The listing builds one solid part. Answer for the finished solid, in the listing's coordinates (mm). Face numbers are marked on the shaded views. Coordinates: 2 decimals unless noted, no trailing zeros. Write each loop counter-clockwise with the first axis right and the second up, starting at its lowest first coordinate (ties: lowest second). Pieces come first, ordered by that corner, then holes. Notation, with made-up numbers: M 17.25,43 L 37.25,43 A15 cw 37.25,62 Z; hole C 54,-27.5 d2. An arc over 180 degrees is marked long. Answer as CSV lines item,"result". Start each with the question number.
```python
from build123d import *

# Parameters (mm, degrees)
F0_R     = 40.88
F0_R_2   = 2.1
F0_R_3   = 40
F1_DEPTH = 2
F2_DEPTH = 10


# Not quite as in the source:
# - a fillet or chamfer that OpenCascade refuses, or shapes differently, is made with other operations: its cross-section is extruded or revolved along the edge and cut away or added


with BuildPart() as f1:
    # F0 (on Top) → F1 (new body)
    with BuildSketch(Plane.XY):
        with BuildLine():
            Line((-41.5, -43), (41.5, -43))
            Line((41.5, -43), (41.5, 43))
            Line((41.5, 43), (-41.5, 43))
            Line((-41.5, 43), (-41.5, 37.85))
            Line((-41.5, 37.85), (-34.75, 37.85))
            ThreePointArc((-34.75, 37.85), (-32.65, 35.75), (-34.75, 33.65))
            Line((-34.75, 33.65), (-41.5, 33.65))
            Line((-41.5, 33.65), (-41.5, -33.65))
            Line((-41.5, -33.65), (-34.75, -33.65))
            ThreePointArc((-34.75, -33.65), (-32.65, -35.75), (-34.75, -37.85))
            Line((-34.75, -37.85), (-41.5, -37.85))
            Line((-41.5, -37.85), (-41.5, -43))
        make_face()
        with BuildLine():
            ThreePointArc((36.75, -33.65), (38.85, -35.75), (36.75, -37.85))
            Line((36.75, -37.85), (31.75, -37.85))
            ThreePointArc((31.75, -37.85), (29.65, -35.75), (31.75, -33.65))
            Line((31.75, -33.65), (36.75, -33.65))
        make_face(mode=Mode.SUBTRACT)
        Circle(F0_R, mode=Mode.SUBTRACT)
        with BuildLine():
            Line((31.75, 37.85), (36.75, 37.85))
            ThreePointArc((36.75, 37.85), (38.85, 35.75), (36.75, 33.65))
            Line((36.75, 33.65), (31.75, 33.65))
            ThreePointArc((31.75, 33.65), (29.65, 35.75), (31.75, 37.85))
        make_face(mode=Mode.SUBTRACT)
        Polygon((41.5, 43), (41.5, -43), (45.5, -43), (45.5, -12), (45.5, 12), (45.5, 43), align=None)
        with BuildLine():
            Line((-124.5, -43), (-41.5, -43))
            Line((-41.5, -43), (-41.5, -37.85))
            Line((-41.5, -37.85), (-48.25, -37.85))
            ThreePointArc((-48.25, -37.85), (-50.35, -35.75), (-48.25, -33.65))
            Line((-48.25, -33.65), (-41.5, -33.65))
            Line((-41.5, -33.65), (-41.5, 33.65))
            Line((-41.5, 33.65), (-48.25, 33.65))
            ThreePointArc((-48.25, 33.65), (-50.35, 35.75), (-48.25, 37.85))
            Line((-48.25, 37.85), (-41.5, 37.85))
            Line((-41.5, 37.85), (-41.5, 43))
            Line((-41.5, 43), (-124.5, 43))
            Line((-124.5, 43), (-124.5, -43))
        make_face()
        with BuildLine():
            Line((-114.75, -37.85), (-119.75, -37.85))
            ThreePointArc((-119.75, -37.85), (-121.85, -35.75), (-119.75, -33.65))
            Line((-119.75, -33.65), (-114.75, -33.65))
            ThreePointArc((-114.75, -33.65), (-112.65, -35.75), (-114.75, -37.85))
        make_face(mode=Mode.SUBTRACT)
        with Locations((-83, 0)):
            Circle(F0_R, mode=Mode.SUBTRACT)
        with BuildLine():
            ThreePointArc((-119.75, 33.65), (-121.85, 35.75), (-119.75, 37.85))
            Line((-119.75, 37.85), (-114.75, 37.85))
            ThreePointArc((-114.75, 37.85), (-112.65, 35.75), (-114.75, 33.65))
            Line((-114.75, 33.65), (-119.75, 33.65))
        make_face(mode=Mode.SUBTRACT)
        Polygon((-128.5, -43), (-124.5, -43), (-124.5, 43), (-128.5, 43), (-128.5, 12), (-128.5, -12), align=None)
        with BuildLine():
            Line((45.5, 12), (45.5, -12))
            ThreePointArc((45.5, -12), (57.5, 0), (45.5, 12))
        make_face()
        with Locations((51.5, 0)):
            Circle(F0_R_2, mode=Mode.SUBTRACT)
        with BuildLine():
            ThreePointArc((-128.5, 12), (-140.5, 0), (-128.5, -12))
            Line((-128.5, -12), (-128.5, 12))
        make_face()
        with Locations((-134.5, 0)):
            Circle(F0_R_2, mode=Mode.SUBTRACT)
        Circle(F0_R)
        Circle(F0_R_3, mode=Mode.SUBTRACT)
        with Locations((-83, 0)):
            Circle(F0_R)
        with Locations((-83, 0)):
            Circle(F0_R_3, mode=Mode.SUBTRACT)
    extrude(amount=F1_DEPTH)

    # F0 (on Top) → F2 (join)
    with BuildSketch(Plane.XY):
        Circle(F0_R)
        Circle(F0_R_3, mode=Mode.SUBTRACT)
        with Locations((-83, 0)):
            Circle(F0_R)
        with Locations((-83, 0)):
            Circle(F0_R_3, mode=Mode.SUBTRACT)
    extrude(amount=F2_DEPTH)

    # F3: fillet of radius 2 on 2 edges, made by hand

    # F3_s1 → F3_t2 (revolve)
    with BuildSketch(Plane.XZ):
        with BuildLine():
            ThreePointArc((-40.12, 2), (-41.5342135624, 2.5857864376), (-42.12, 4))
            Line((-42.12, 4), (-42.12, 2))
            Line((-42.12, 2), (-40.12, 2))
        make_face()
    revolve(axis=Axis((-83, 0, 2), (0, 0, -1)))

    # F3_s3 → F3_t4 (revolve)
    with BuildSketch(Plane.XZ):
        with BuildLine():
            ThreePointArc((42.88, 2), (41.4657864376, 2.5857864376), (40.88, 4))
            Line((40.88, 4), (40.88, 2))
            Line((40.88, 2), (42.88, 2))
        make_face()
    revolve(axis=Axis((0, 0, 2), (0, 0, -1)))


solid = f1.part
```
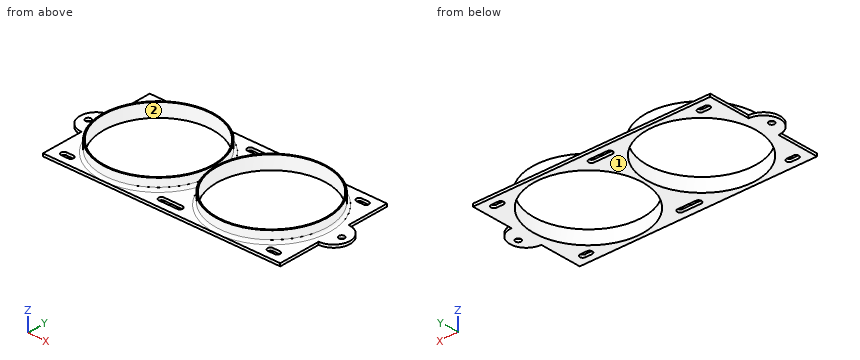
1) Find the intervals of material crossed by line 1 (X direction, y = 1.5, z = 7.75); line 2 (X direction, y = 1.5, z = 1); line 3 (X direction, y = -34, z = 5.5), in increasing order. Write a range as from..to.
2) Each of these flat-tipped pins is pushed along its axis until it touches: P1, Ø2, axis at x = -53.5, z = 5.5, coming from the -Y side; P2, Ø5, axis at y = -20, z = 1.5, coming from the -X side; P3, Ø6, axis at x = -94, z = 6.5, coming from the +Y side. Where does it stop, or does it pass through?
3) The part is cut by section B-B (x = -134.5). Determine the outline of the cut face in (y, z).
4) The part is cut by section A-A (z = 7.5). Determine the outline of the cut face in (x, y), then the cut area to 3 significant figures.
5) The part is cut by section C-C (y = 0). Count the separate pieces of the cut face and the enclosed holes in it, then the cut area to 3 significant figures.
6) For a pull along Y with two mould halves and no side action, classify the marked faces 1 and 2 as +Y half, -Y half, draft (parallel to the pull), parting line (faces both ways), or undercut.
Completed:
1,line 1,"-123.85..-122.97, -43.03..-42.15, -40.85..-39.97, 39.97..40.85"
1,line 2,"-140.41..-135.97, -133.03..-122.97, -43.03..-39.97, 39.97..50.03, 52.97..57.41"
1,line 3,"-105.7..-104.07, -61.93..-60.3, -22.7..-21.07, 21.07..22.7"
2,P1,"y = -29.31"
2,P2,"x = -128.5"
2,P3,"y = 40.09"
3,outline,"M -10.39,0 L -2.1,0 L -2.1,2 L -10.39,2 Z; M 2.1,0 L 10.39,0 L 10.39,2 L 2.1,2 Z"
4,outline,"C -83,0 d81.76; C 0,0 d81.76; hole C -83,0 d80; hole C 0,0 d80"
4,area,"447 mm²"
5,separate pieces,"5"
5,enclosed holes,"0"
5,area,"90.3 mm²"
6,face 1,"draft"
6,face 2,"undercut"
